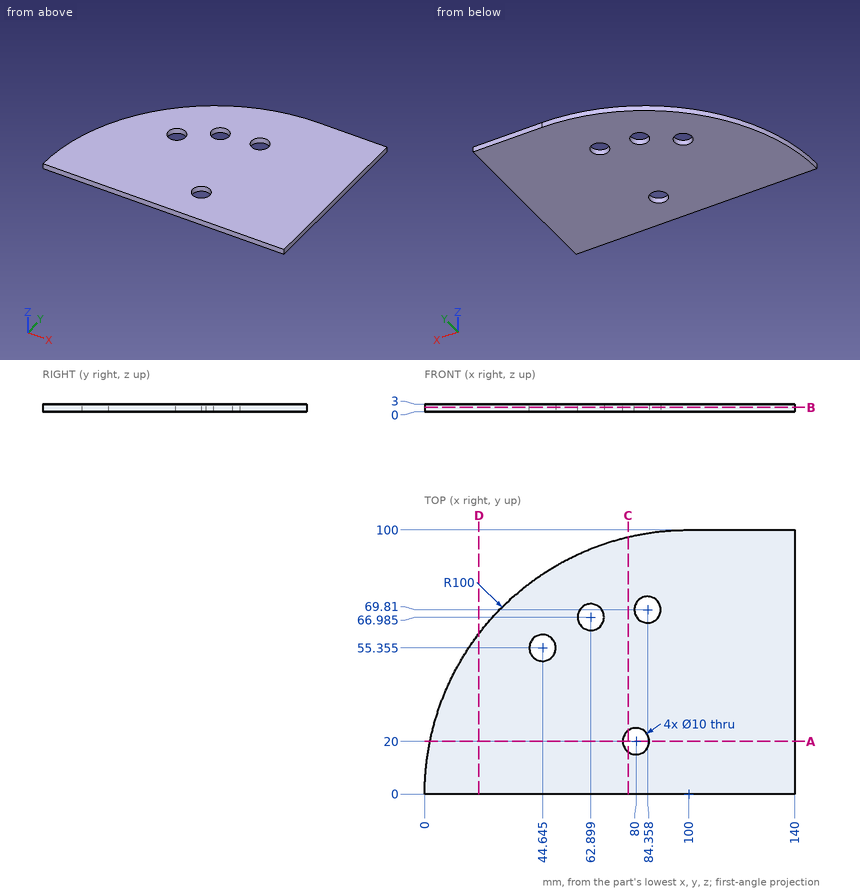
Drawing for the job (mm, zero at the part's lowest x, y, z). Round coordinates to 2 decimals unless told otherwise and drop trailing zeros. Loops run counter-clockwise (first coordinate to the right, second up) from the corner with the lowest first, then second, coordinate; pieces in that order, holes last. Notation, with made-up numbers: (79.5, 26.5) -> (98.5, 26.5) arc R19 ccw to (98.5, 52.5) -> close; hole circle Ø2 at (23, -1.5). An arc over 180 degrees is marked (long way). Answer in a Markdown table with one row per item.
Item 1: Saw through at C-C (x = 77). Write the cut outline in (y, z), and give its area (3 significant figures).
Answers below:
| item | result |
|---|---|
| outline | (0, 0) -> (16, 0) -> (16, 3) -> (0, 3) -> close; (24, 0) -> (97.32, 0) -> (97.32, 3) -> (24, 3) -> close |
| area | 268 mm² |
Item 2: Saw through at A-A (y = 20). Write the cut outline in (x, z).
Answers below:
| item | result |
|---|---|
| outline | (2.02, 0) -> (75, 0) -> (75, 3) -> (2.02, 3) -> close; (85, 0) -> (140, 0) -> (140, 3) -> (85, 3) -> close |
Item 3: Drill centre lines: L1, parallel to X at y = 66.5, z = 0.45 (1 decimal); L2, parallel to Y at x = 62, z = 1.7 (1 decimal); L3, parallel to Y at x = 80, z = 0.8 (1 decimal). Where is each one in solid material? Low to high. Write a range as [from, to].
Answers below:
| item | result |
|---|---|
| L1 | x = [25.3, 57.9], [67.9, 80.6], [88.1, 140] |
| L2 | y = [0, 62.1], [71.9, 92.5] |
| L3 | y = [0, 15], [25, 67.4], [72.3, 98] |
Item 4: Saw through at B-B (z = 1.7). Write the cut outline in (x, y) (1 decimal), and give its area (3 significant figures).
Answers below:
| item | result |
|---|---|
| outline | (0, 0) -> (140, 0) -> (140, 100) -> (100, 100) arc R100 ccw to start; hole circle Ø10 at (44.6, 55.4); hole circle Ø10 at (62.9, 67); hole circle Ø10 at (80, 20); hole circle Ø10 at (84.4, 69.8) |
| area | 11,500 mm² |
Item 5: Pin check, flat tips, straight feed: pin 1 (13 mm diameter, centred on x = 62.9, y = 66.98, fed in from -Z); pin 2 (1.5 mm diameter, centred on y = 12.5, z = 1.5, fed in from -X). Stop position of each tip, or through.
Answers below:
| item | result |
|---|---|
| pin 1 | stops at z = 0 |
| pin 2 | stops at x = 0.69 |
Item 6: Saw through at D-D (x = 20.5). Write the cut outline in (y, z).
Answers below:
| item | result |
|---|---|
| outline | (0, 0) -> (60.66, 0) -> (60.66, 3) -> (0, 3) -> close |
